```python
from build123d import *

# Parameters (mm, degrees)
SKETCH1_W               = 505
SKETCH1_H               = 500
SKETCH1_W_2             = 499
SKETCH1_H_2             = 494
BOSS_EXTRUDE1_DEPTH     = 500
CUT_EXTRUDE2_DEPTH      = 751.837032917
CUT_EXTRUDE2_DEPTH_BACK = 751.837032917
SKETCH4_R               = 4
SKETCH4_R_2             = 2.5


with BuildPart() as part:
    # Sketch1 → Boss-Extrude1 (new body)
    with BuildSketch(Plane(origin=(0, 0, 0), x_dir=(1, 0, 0), z_dir=(0, 1, 0))):
        Rectangle(SKETCH1_W, SKETCH1_H)
        Rectangle(SKETCH1_W_2, SKETCH1_H_2, mode=Mode.SUBTRACT)
    extrude(amount=BOSS_EXTRUDE1_DEPTH)

    # Sketch4 → Cut-Extrude2 (cut, two sides: drawn at the far end of the back side and taken through both)
    with BuildSketch(Plane(origin=(0, 0, -250), x_dir=(-1, 0, 0), z_dir=(0, 0, -1)).offset(-CUT_EXTRUDE2_DEPTH_BACK)):
        with Locations((35, 400)):
            Circle(SKETCH4_R)
        with Locations(Location((-35, 400, 0), (0, 0, 180))):
            Circle(SKETCH4_R)
        with Locations((-19, 400)):
            Circle(SKETCH4_R_2)
        with Locations(Location((-51, 400, 0), (0, 0, 180))):
            Circle(SKETCH4_R_2)
        with Locations(Location((19, 400, 0), (0, 0, 180))):
            Circle(SKETCH4_R_2)
        with Locations((51, 400)):
            Circle(SKETCH4_R_2)
    extrude(amount=CUT_EXTRUDE2_DEPTH + CUT_EXTRUDE2_DEPTH_BACK, mode=Mode.SUBTRACT)


solid = part.part
```
For this review, take the finished solid that the model builds, in its own axes (mm). A direction names the side the tool comes from. Round coordinates to 2 decimals unless told otherwise and drop trailing zeros. Loops run counter-clockwise (first coordinate to the right, second up) from the corner with the lowest first, then second, coordinate; pieces in that order, holes last.
Q1. To check wall thickness, follow line 1 along X through (y, z) = (140.5, -213.5); line 2 along Z through (x, y) = (-187.5, 141.5); line 3 along Y through (x, z) = (-35, -249). State the ranges of each line that lie inside material, in increasing order.
Result sheet:
line 1: x = -252.5 to -249.5, 249.5 to 252.5
line 2: z = -250 to -247, 247 to 250
line 3: y = 0 to 396, 404 to 500
Q2. Insertion check: pin 1 Ø6.5 at (x, y) = (-35, 400) entering from -Z. The pin has a flat end and moves straight along its axis. Give the tip position at first contact, or say it passes through.
Result sheet:
pin 1: passes through
Q3. Add section A-A on x = 176.5. Write out the cut boundary in (y, z).
Result sheet:
outline: (0, -250) - (500, -250) - (500, -247) - (0, -247) - close; (0, 247) - (500, 247) - (500, 250) - (0, 250) - close
Q4. Add section B-B on z = 190.5. Write out the cut boundary in (x, y).
Result sheet:
outline: (-252.5, 0) - (-249.5, 0) - (-249.5, 500) - (-252.5, 500) - close; (249.5, 0) - (252.5, 0) - (252.5, 500) - (249.5, 500) - close
Q5. Mouldability with a two-part tool opening along Z and no side actions: class faces 1 (the face through (-4, 246, -250)), 2 (the face through (249.5, 246, 3)), 3 (the face through (-4, 246, 250)), 4 (the face through (-252.5, 246, 3)) as +Z half, -Z half, draft (parallel to the pull), parting line (faces both ways), or undercut.
Result sheet:
face 1: -Z half
face 2: undercut
face 3: +Z half
face 4: draft
Q6. Machinability: for faces 5 (the face through (252.5, 246, 3)), 6 (the face through (-3, 246, 247)), which of the approach directions +Z, -Z, +X, -X, +Y, -Y give a long, thin tool a straight path to every point of the face, cutting with its end or side? Answer none if there is none.
Result sheet:
face 5: +Z, -Z, +X, +Y, -Y
face 6: +Y, -Y
Q7. Add section C-C on y = 199. Write out the cut boundary in (x, z), plus the area to 3 significant figures.
Result sheet:
outline: (-252.5, -250) - (252.5, -250) - (252.5, 250) - (-252.5, 250) - close; hole (-249.5, -247) - (249.5, -247) - (249.5, 247) - (-249.5, 247) - close
area: 5,990 mm2
